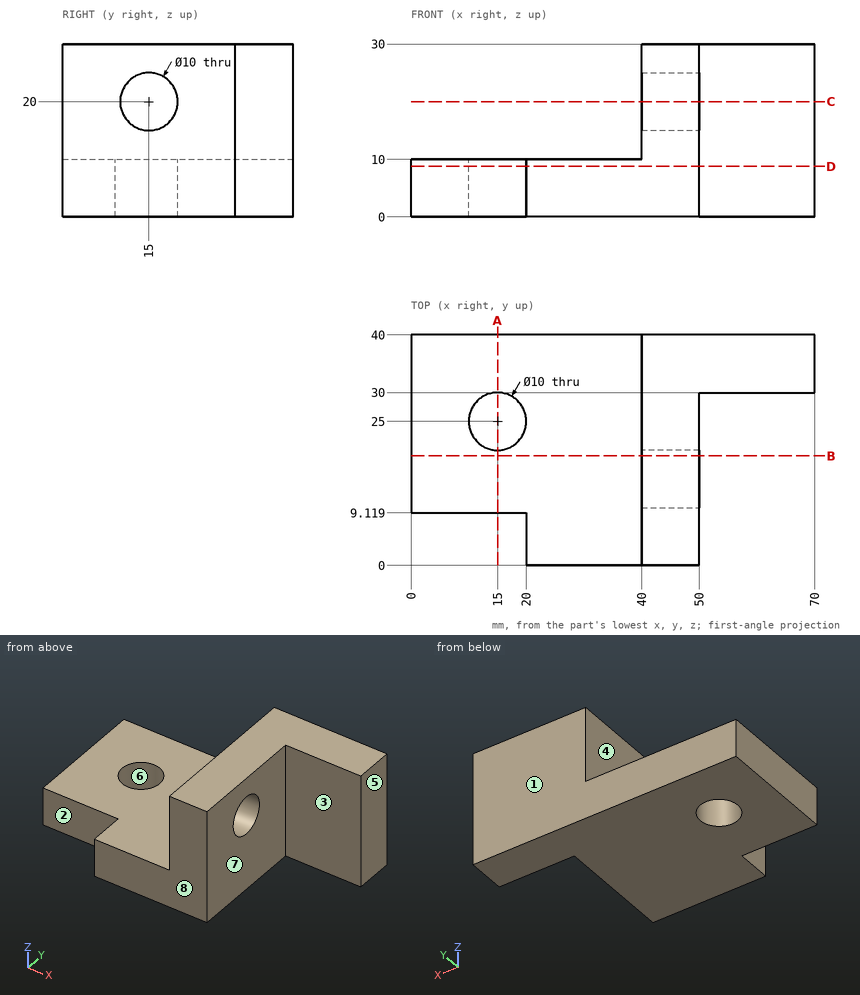
Part print with two shaded views. Sizes in mm from the minimum x, y, z corner. A direction names the side the tool comes from. Round coordinates to 2 decimals unless told otherwise and drop trailing zeros. Loops run counter-clockwise (first coordinate to the right, second up) from the corner with the lowest first, then second, coordinate; pieces in that order, holes last. Notation, with made-up numbers: M 15.25,19.25 L 60.25,19.25 A34 ccw 60.25,55.25 Z; hole C 48,17 d8. An arc over 180 degrees is marked long. Put each result on its own line as item: value. Start each with the question number.
Item 1: Cut at D-D (z = 8.75). List the corners of the cut face in (x, y).
Item 2: Drill centre lines: line 1 along Z through (x, y) = (47, 15); line 2 along Y through (x, z) = (15, 5.5); line 3 along Z through (x, y) = (6.5, 30). Where is each one in solid material? Low to high.
Item 3: Cut at A-A (x = 15). List the corners of the cut face in (y, z), then the cut area to 3 significant figures.
Item 4: Cut at C-C (z = 20). List the corners of the cut face in (x, y).
Item 5: 3-axis set-ups, long thin cutter, end or side, ignore diameter. For the marked faces 1, 2, 3, 4 and 5: which of +Z, -Z, +X, -X, +Y, -Y reach the whole face in a straight line?
Item 6: Mould opens along Y. For the marked faces 6, 7 and 8 say: released by +Y, released by -Y, zero draft, split by the parting line, or undercut.
Item 7: Drop flat-ended pins along their axis: P1, Ø10, axis at y = 17, z = 20.5, coming from the -X side; P2, Ø13, axis at x = 15, y = 25, coming from the +Z side; P3, Ø4.5, axis at y = 3, z = 7.5, coming from the -X side. Give the stop position or say it passes through.
Item 8: Cut at B-B (y = 19). List the corners of the cut face in (x, z), then the cut area to 3 significant figures.
Answer block:
1. outline: M 0,9.12 L 20,9.12 L 20,0 L 50,0 L 50,30 L 70,30 L 70,40 L 0,40 Z; hole C 15,25 d10
2. line 1: 0 to 15, 25 to 30
2. line 2: 9.12 to 20, 30 to 40
2. line 3: 0 to 10
3. outline: M 9.12,0 L 20,0 L 20,10 L 9.12,10 Z; M 30,0 L 40,0 L 40,10 L 30,10 Z
3. area: 209 mm2
4. outline: M 40,0 L 50,0 L 50,10 L 40,10 Z; M 40,20 L 50,20 L 50,30 L 70,30 L 70,40 L 40,40 Z
5. face 1: +Z, -Z, +X, -X, +Y
5. face 2: +Z, -Z, -X, -Y
5. face 3: +Z, -Z, +X, -Y
5. face 4: +Z, -X, +Y, -Y
5. face 5: +Z, -Z, +X, +Y, -Y
6. face 6: undercut
6. face 7: zero draft
6. face 8: released by -Y
7. P1: x = 40
7. P2: z = 10
7. P3: x = 20
8. outline: M 0,0 L 50,0 L 50,17 L 40,17 L 40,10 L 0,10 Z; M 40,23 L 50,23 L 50,30 L 40,30 Z
8. area: 640 mm2
